from build123d import *

# Parameters (mm, degrees)
SKETCH1_W           = 114.3
SKETCH1_H           = 2.9972
BOSS_EXTRUDE1_DEPTH = 2.9972
SKETCH2_R           = 1.397
CUT_EXTRUDE1_DEPTH  = 3.9972
SKETCH3_W           = 25.4
SKETCH3_H           = 2.9972
BOSS_EXTRUDE2_DEPTH = 2.9972
SKETCH4_W           = 155.8544
SKETCH4_H           = 0.762
BOSS_EXTRUDE3_DEPTH = 2.9972
SKETCH5_R           = 1.397
CUT_EXTRUDE2_DEPTH  = 3.9972
SKETCH7_R           = 1.397
CUT_EXTRUDE3_DEPTH  = 3.9972
SKETCH6_W           = 25.4
SKETCH6_H           = 6.096
CUT_EXTRUDE4_DEPTH  = 3.9972


with BuildPart() as part:
    # Sketch1 → Boss-Extrude1 (new body)
    with BuildSketch(Plane.XY):
        Polygon((139.7, 23.9268), (139.7, 0), (147.7772, 0), (147.7772, 47.8536), (142.6972, 47.8536), (142.6972, 23.9268), align=None)
        Polygon((0, 23.9268), (0, 0), (139.7, 0), (139.7, 23.9268), (139.7, 47.8536), (127, 47.8536), (127, 44.8564), (12.7, 44.8564), (12.7, 47.8536), (0, 47.8536), align=None)
        with Locations((69.85, 7.8486)):
            Rectangle(SKETCH1_W, SKETCH1_H, mode=Mode.SUBTRACT)
        with Locations((69.85, 33.1978)):
            Rectangle(SKETCH1_W, SKETCH1_H, mode=Mode.SUBTRACT)
        Polygon((-8.0772, 0), (0, 0), (0, 23.9268), (-2.9972, 23.9268), (-2.9972, 47.8536), (-8.0772, 47.8536), align=None)
    extrude(amount=BOSS_EXTRUDE1_DEPTH)

    # Sketch2 → Cut-Extrude1 (cut, through all)
    with BuildSketch(Plane(origin=(0, 0, 0), x_dir=(-1, 0, 0), z_dir=(0, 0, -1))):
        with Locations((-108.1024, 12.6492)):
            Circle(SKETCH2_R)
        with Locations((-31.5976, 12.6492)):
            Circle(SKETCH2_R)
        with Locations((-108.1024, 37.9984)):
            Circle(SKETCH2_R)
        with Locations((-31.5976, 37.9984)):
            Circle(SKETCH2_R)
    extrude(amount=-CUT_EXTRUDE1_DEPTH, mode=Mode.SUBTRACT)

    # Sketch3 → Boss-Extrude2 (add)
    with BuildSketch(Plane(origin=(0, 0, 0), x_dir=(-1, 0, 0), z_dir=(0, 0, -1))):
        with Locations((-114.3, 46.355)):
            Rectangle(SKETCH3_W, SKETCH3_H)
        with Locations((-114.3, 33.1978)):
            Rectangle(SKETCH3_W, SKETCH3_H)
        with Locations((-114.3, 7.8486)):
            Rectangle(SKETCH3_W, SKETCH3_H)
        with Locations((-25.4, 7.8486)):
            Rectangle(SKETCH3_W, SKETCH3_H)
        with Locations((-25.4, 33.1978)):
            Rectangle(SKETCH3_W, SKETCH3_H)
        with Locations((-25.4, 46.355)):
            Rectangle(SKETCH3_W, SKETCH3_H)
    extrude(amount=-BOSS_EXTRUDE2_DEPTH)

    # Sketch4 → Boss-Extrude3 (add)
    with BuildSketch(Plane(origin=(0, 0, 0), x_dir=(-1, 0, 0), z_dir=(0, 0, -1))):
        with Locations((-69.85, -0.381)):
            Rectangle(SKETCH4_W, SKETCH4_H)
    extrude(amount=-BOSS_EXTRUDE3_DEPTH)

    # Sketch5 → Cut-Extrude2 (cut, through all)
    with BuildSketch(Plane.XY.offset(2.9972)):
        with Locations((31.5976, 28.3972)):
            Circle(SKETCH5_R)
        with Locations((108.1024, 28.3972)):
            Circle(SKETCH5_R)
    extrude(amount=-CUT_EXTRUDE2_DEPTH, mode=Mode.SUBTRACT)

    # Sketch7 → Cut-Extrude3 (cut, through all)
    with BuildSketch(Plane(origin=(0, 0, 0), x_dir=(-1, 0, 0), z_dir=(0, 0, -1))):
        with Locations((-108.1024, 3.048)):
            Circle(SKETCH7_R)
        with Locations((-31.5976, 3.048)):
            Circle(SKETCH7_R)
    extrude(amount=-CUT_EXTRUDE3_DEPTH, mode=Mode.SUBTRACT)

    # Sketch6 → Cut-Extrude4 (cut, through all)
    with BuildSketch(Plane.XY.offset(2.9972)):
        with Locations((34.036, 22.0472)):
            Rectangle(SKETCH6_W, SKETCH6_H)
        with Locations((105.664, 22.0472)):
            Rectangle(SKETCH6_W, SKETCH6_H)
    extrude(amount=-CUT_EXTRUDE4_DEPTH, mode=Mode.SUBTRACT)


solid = part.part
Build history of the part. All positions in model axes, mm. A direction names the side the tool comes from. Coordinates: 2 decimals unless noted, no trailing zeros. Order: outer loops, then holes, each group sorted by start corner. A loop starts at its lowest first (then second) coordinate and runs counter-clockwise, first axis right, second up. Notation, with made-up numbers: (5.25, -31.75) - (26.25, -31.75) arc R22 cw to (26.25, -3.75) - close; hole circle Ø2 at (20, 39.5). An arc over 180 degrees is marked (long way). Put each result on its own line as item: value.
1. Tool access for faces 1 (the face through (-1, 23.927, 1)), 2 (the face through (46.736, 22, 2)), 3 (the face through (71, -0.762, 1)): list every direction of +Z, -Z, +X, -X, +Y, -Y with a clear straight run to the whole face (end or side of a thin tool).
Answer sheet:
face 1: +Z, -Z, +Y
face 2: +Z, -Z
face 3: +Z, -Z, +X, -X, -Y
2. Saw through at C-C (x = 104.5). Write the cut outline in (y, z).
Answer sheet:
outline: (-0.76, 0) - (19, 0) - (19, 3) - (-0.76, 3) - close; (25.1, 0) - (47.85, 0) - (47.85, 3) - (25.1, 3) - close
3. Saw through at B-B (y = 42). Write the cut outline in (x, z), and give its area (3 significant figures).
Answer sheet:
outline: (-8.08, 0) - (-3, 0) - (-3, 3) - (-8.08, 3) - close; (0, 0) - (139.7, 0) - (139.7, 3) - (0, 3) - close; (142.7, 0) - (147.78, 0) - (147.78, 3) - (142.7, 3) - close
area: 449 mm^2
4. Pull direction X, two halves, no side cores. Call faces 4 (the face through (-6, 47.854, 1)), 5 (the face through (70, 44.856, 1)): pulls with the +X half, pulls with the -X half, needs draft (parallel to the pull), parting line crosses it, or undercut.
Answer sheet:
face 4: needs draft
face 5: undercut
5. Saw through at A-A (x = 65). Write the cut outline in (y, z), and give its area (3 significant figures).
Answer sheet:
outline: (-0.76, 0) - (6.35, 0) - (6.35, 3) - (-0.76, 3) - close; (9.35, 0) - (31.7, 0) - (31.7, 3) - (9.35, 3) - close; (34.7, 0) - (44.86, 0) - (44.86, 3) - (34.7, 3) - close
area: 119 mm^2
6. Probe line 1 along Y through (x, z) = (43, 1.1); line 2 along X through (y, z) = (43, 2.7); line 3 along X through (y, z) = (23, 2.2). List the from-to ranges inside material, lowest first. Write a range as [from, to].
Answer sheet:
line 1: y = [-0.76, 6.35], [9.35, 19], [25.1, 31.7], [34.7, 44.86]
line 2: x = [-8.08, -3], [0, 139.7], [142.7, 147.78]
line 3: x = [-8.08, 21.34], [46.74, 92.96], [118.36, 147.78]
7. Saw through at D-D (x = 40). Write the cut outline in (y, z).
Answer sheet:
outline: (-0.76, 0) - (6.35, 0) - (6.35, 3) - (-0.76, 3) - close; (9.35, 0) - (19, 0) - (19, 3) - (9.35, 3) - close; (25.1, 0) - (31.7, 0) - (31.7, 3) - (25.1, 3) - close; (34.7, 0) - (44.86, 0) - (44.86, 3) - (34.7, 3) - close
8. Drop flat-ended pins along their axis: P1, Ø3, axis at x = 31.6, y = 38, coming from the +Z side; P2, Ø1.5, axis at x = 140.5, z = 1, coming from the +Y side; P3, Ø1.5, axis at x = 77.5, z = 1, coming from the +Y side. Give the stop position or say it passes through.
Answer sheet:
P1: stops at z = 3
P2: stops at y = 23.93
P3: stops at y = 44.86
